```python
from build123d import *

# Parameters (mm, degrees)
BOSS_EXTRUDE2_DEPTH        = 5
SKETCH2_R                  = 9.525
BOSS_EXTRUDE3_DEPTH        = 33.1
SKETCH3_R                  = 3.96875
CUT_EXTRUDE1_DEPTH         = 19.05
SKETCH4_R                  = 1.27
CUT_EXTRUDE2_DEPTH         = 19.05
F_10_24_TAPPED_HOLE1_D     = 3.7973
F_10_24_TAPPED_HOLE1_DEPTH = 14.95
F_10_24_TAPPED_HOLE1_TIP   = 1.140824014
SKETCH6_R                  = 1.27
CUT_EXTRUDE3_DEPTH         = 8


with BuildPart() as part:
    # Sketch1 → Boss-Extrude2 (new body)
    with BuildSketch(Plane.XY):
        Polygon((0, 8.082903769), (-7, 4.041451884), (-7, -4.041451884), (0, -8.082903769), (7, -4.041451884), (7, 4.041451884), align=None)
    extrude(amount=BOSS_EXTRUDE2_DEPTH)

    # Sketch2 → Boss-Extrude3 (add)
    with BuildSketch(Plane(origin=(0, 0, 0), x_dir=(-1, 0, 0), z_dir=(0, 0, -1))):
        Circle(SKETCH2_R)
    extrude(amount=BOSS_EXTRUDE3_DEPTH)

    # Sketch3 → Cut-Extrude1 (cut)
    with BuildSketch(Plane(origin=(0, 0, -33.1), x_dir=(-1, 0, 0), z_dir=(0, 0, -1))):
        Circle(SKETCH3_R)
    extrude(amount=-CUT_EXTRUDE1_DEPTH, mode=Mode.SUBTRACT)

    # Sketch4 → Cut-Extrude2 (cut)
    with BuildSketch(Plane.XY.offset(5)):
        Circle(SKETCH4_R)
    extrude(amount=-CUT_EXTRUDE2_DEPTH, mode=Mode.SUBTRACT)

    # #10-24 Tapped Hole1
    with Locations(Plane.XY.offset(5)):
        with Locations((0, 0)):
            Hole(F_10_24_TAPPED_HOLE1_D / 2, depth=F_10_24_TAPPED_HOLE1_DEPTH)
            with Locations((0, 0, -(F_10_24_TAPPED_HOLE1_DEPTH + F_10_24_TAPPED_HOLE1_TIP / 2))):  # 118° drill point
                Cone(0, F_10_24_TAPPED_HOLE1_D / 2, F_10_24_TAPPED_HOLE1_TIP, mode=Mode.SUBTRACT)

    # Sketch6 → Cut-Extrude3 (cut)
    with BuildSketch(Plane(origin=(9.525, 0, 0), x_dir=(0, 0, -1), z_dir=(1, 0, 0))):
        with Locations((13.755140778, 0)):
            Circle(SKETCH6_R)
    extrude(amount=-CUT_EXTRUDE3_DEPTH, mode=Mode.SUBTRACT)


solid = part.part
```
CAD build for the part. Positions are in the model's coordinates, mm. A direction names the side the tool comes from. Round coordinates to 2 decimals unless told otherwise and drop trailing zeros. Order: outer loops, then holes, each group sorted by start corner. A loop starts at its lowest first (then second) coordinate and runs counter-clockwise, first axis right, second up. Notation, with made-up numbers: (83.25, -1.5) -> (126.25, -1.5) arc R32 cw to (126.25, 35.5) -> close; hole circle Ø8 at (22.5, 77). An arc over 180 degrees is marked (long way). Write item = value, one per line.
(1) Flat gauge pins, fed straight in: P1, Ø8, axis at x = -7.5, y = 6, coming from the +Z side; P2, Ø4, axis at y = 0.5, z = 3.5, coming from the -X side; P3, Ø1.5, axis at y = -4, z = -25, coming from the -X side; P4, Ø4, axis at y = -5.5, z = -15.5, coming from the +X side. Where does each tip first touch, or does it go through?
Answers follow:
P1 = 5
P2 = -7
P3 = -8.95
P4 = 8.86
(2) 3-axis set-ups, long thin cutter, end or side, ignore diameter. For faces 1 (the cylindrical face through (0.86, -3.874, -23.708)), 2 (the flat face through (4, -6, 0)), 3 (the flat face through (7, 0, 2)): which of +Z, -Z, +X, -X, +Y, -Y reach the whole face in a straight line?
Answers follow:
face_1 = -Z
face_2 = +Z
face_3 = +Z, +X, +Y, -Y
(3) Pull direction Y, two halves, no side cores. Call faces 4 (the flat face through (-3.549, -6.034, 2.465)), 5 (the flat face through (-4, -2, -33.1)), 6 (the cylindrical face through (6.47, 0.056, -12.486)): +Y half, -Y half, draft (parallel to the pull), parting line (faces both ways), or undercut.
Answers follow:
face_4 = -Y half
face_5 = draft
face_6 = undercut
(4) Cut at A-A (y = 0). Write the cut outline in (x, z) (3 decimals).
Answers follow:
outline = (-9.525, -33.1) -> (-3.969, -33.1) -> (-3.969, -14.05) -> (-1.27, -14.05) -> (-1.27, -10.328) -> (-1.899, -9.95) -> (-1.899, 5) -> (-7, 5) -> (-7, 0) -> (-9.525, 0) -> close; (1.27, -14.05) -> (1.525, -14.05) -> (1.525, -12.485) -> (9.525, -12.485) -> (9.525, 0) -> (7, 0) -> (7, 5) -> (1.899, 5) -> (1.899, -9.95) -> (1.27, -10.328) -> close; (3.969, -33.1) -> (9.525, -33.1) -> (9.525, -15.025) -> (3.969, -15.025) -> close
(5) Cut at D-D (x = -3.5). Write the cut outline in (y, z).
Answers follow:
outline = (-8.86, -33.1) -> (-1.87, -33.1) -> (-1.87, -14.05) -> (1.87, -14.05) -> (1.87, -33.1) -> (8.86, -33.1) -> (8.86, 0) -> (6.06, 0) -> (6.06, 5) -> (-6.06, 5) -> (-6.06, 0) -> (-8.86, 0) -> close
(6) Cut at C-C (z = -8.5). Write the cut outline in (x, y) (3 decimals).
Answers follow:
outline = circle Ø19.05 at (0, 0); hole circle Ø3.797 at (0, 0)
(7) Drill centre lines: L1, parallel to Y at x = 0, z = -5 (3 decimals); L2, parallel to X at y = 0, z = 1.25; L3, parallel to X at y = 0, z = -21 (3 decimals). Where is each one in solid material? Low to high.
Answers follow:
L1 = -9.525 to -1.899, 1.899 to 9.525
L2 = -7 to -1.9, 1.9 to 7
L3 = -9.525 to -3.969, 3.969 to 9.525
(8) Cut at B-B (x = 6.5). Write the cut outline in (y, z), plus the area to 3 significant figures.
Answers follow:
outline = (-6.96, -33.1) -> (6.96, -33.1) -> (6.96, 0) -> (4.33, 0) -> (4.33, 5) -> (-4.33, 5) -> (-4.33, 0) -> (-6.96, 0) -> close; hole circle Ø2.54 at (0, -13.76)
area = 499 mm²
